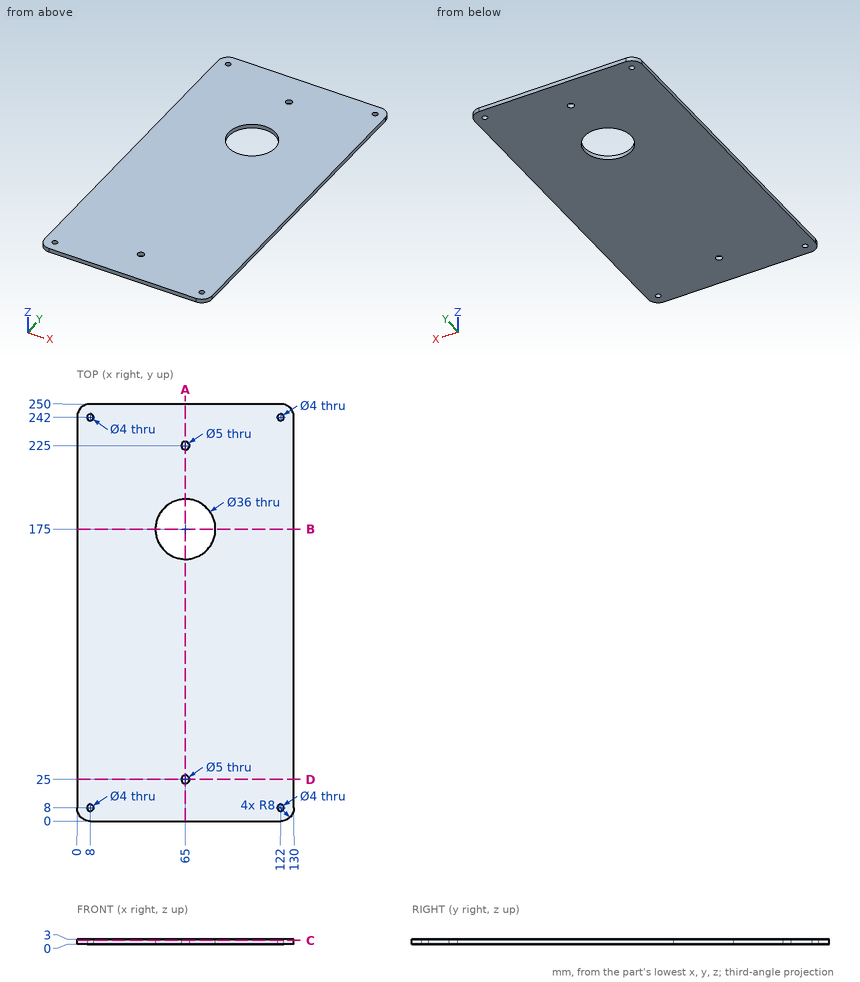
Geometry: see drawing. Coordinates: mm, zero at the bounding-box minimum. Give positions to 0.01 mm unless a question says otherwise; leave off trailing zeros. Order: outer loops, then holes, each group sorted by start corner. A loop starts at its lowest first (then second) coordinate and runs counter-clockwise, first axis right, second up. Notation, with made-up numbers: M 18.25,86.25 L 45.25,86.25 A9 cw 45.25,96.25 Z; hole C 83.5,6 d9. An arc over 180 degrees is marked long. Answer as CSV lines item,"result". Start each with the question number.
1) Cut plane C-C (z = 2.2). Output: boundary loops of the cut face in (x, y).
2) Cut plane D-D (y = 25). Output: boundary loops of the cut face in (x, z).
3) Cut plane A-A (x = 65). Output: boundary loops of the cut face in (y, z), then the cut area to 3 significant figures.
4) Cut plane B-B (y = 175). Output: boundary loops of the cut face in (x, z), then the cut area to 3 significant figures.
5) Line query: line 1 (Y direction, x = 8, z = 0.8); line 2 (X direction, y = 242, z = 2.35); line 3 (Y direction, x = 65, z = 2.2). Output: solid intervals per line, ascending. Write a range as from..to.
6) First-contact query: P1, Ø3, axis at x = 65, y = 25, coming from the -Z side; P2, Ø3, axis at x = 107, y = 162, coming from the -Z side. Flat tips, straight axial feed; report the tip coordinate or a pass-through.
Findings below:
1,outline,"M 0,8 A8 ccw 8,0 L 122,0 A8 ccw 130,8 L 130,242 A8 ccw 122,250 L 8,250 A8 ccw 0,242 Z; hole C 8,8 d4; hole C 8,242 d4; hole C 65,175 d36; hole C 65,25 d5; hole C 65,225 d5; hole C 122,8 d4; hole C 122,242 d4"
2,outline,"M 0,0 L 62.5,0 L 62.5,3 L 0,3 Z; M 67.5,0 L 130,0 L 130,3 L 67.5,3 Z"
3,outline,"M 0,0 L 22.5,0 L 22.5,3 L 0,3 Z; M 27.5,0 L 157,0 L 157,3 L 27.5,3 Z; M 193,0 L 222.5,0 L 222.5,3 L 193,3 Z; M 227.5,0 L 250,0 L 250,3 L 227.5,3 Z"
3,area,"612 mm²"
4,outline,"M 0,0 L 47,0 L 47,3 L 0,3 Z; M 83,0 L 130,0 L 130,3 L 83,3 Z"
4,area,"282 mm²"
5,line 1,"y = 0..6, 10..240, 244..250"
5,line 2,"x = 0..6, 10..120, 124..130"
5,line 3,"y = 0..22.5, 27.5..157, 193..222.5, 227.5..250"
6,P1,"passes through"
6,P2,"stops at z = 0"
